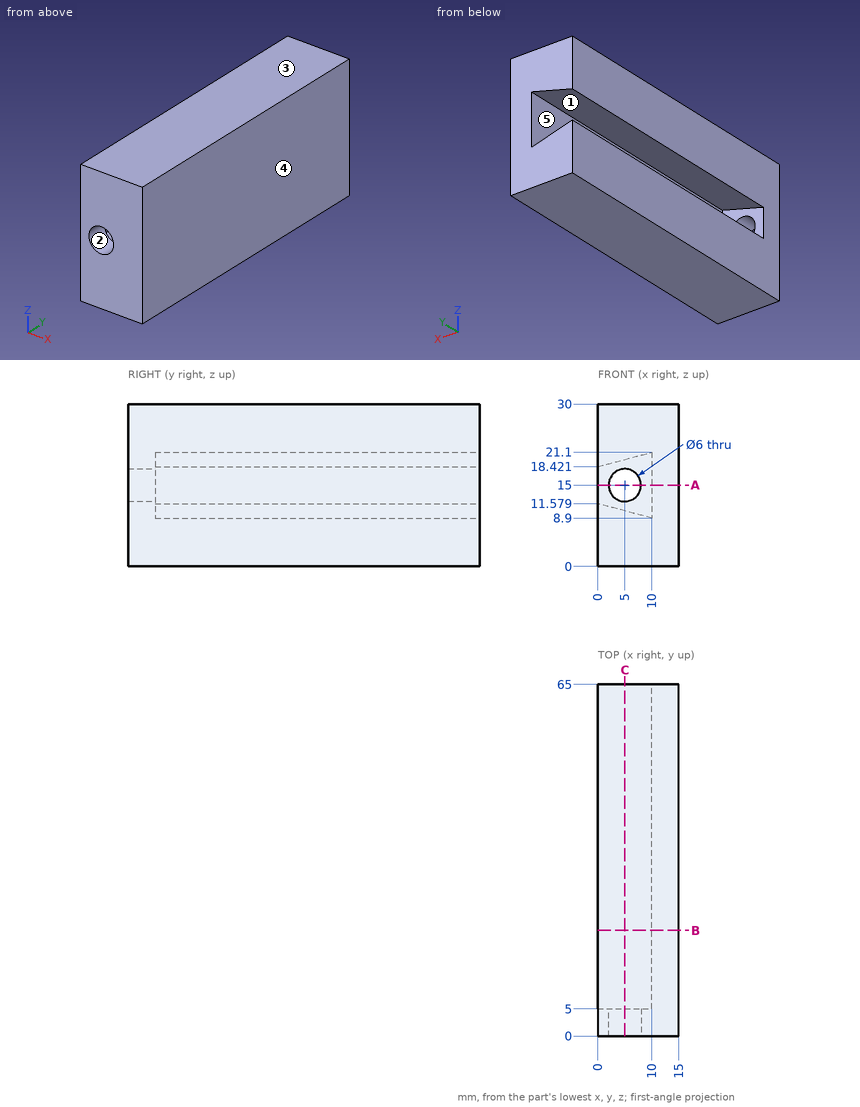
Study the drawing (mm; zero at the part's minimum x, y, z) and answer. A direction names the side the tool comes from. Give positions to 0.01 mm unless a question says otherwise; leave off trailing zeros. Write each loop counter-clockwise with the first axis right and the second up, starting at its lowest first coordinate (ties: lowest second). Pieces come first, ordered by that corner, then holes. Notation, with made-up numbers: (50, 88.5) -> (95, 88.5) arc R20 cw to (95, 126.5) -> close; hole circle Ø11 at (72.25, 85). An arc over 180 degrees is marked (long way). Write item = value, one per line.
Q1. A flat-ended cylindrical pin translates along its axis: pin 1 Ø8 at (y, z) = (49.5, 21.5) entering from -X. Find the tip coordinate at first contact, or state that the pin passes through.
Computed values:
pin_1 = 0
Q2. Section B-B on y = 19.5 is taken. Determine the outline of the cut face in (x, z), and give its area (3 significant figures).
Computed values:
outline = (0, 0) -> (15, 0) -> (15, 30) -> (0, 30) -> (0, 18.42) -> (10, 21.1) -> (10, 8.9) -> (0, 11.58) -> close
area = 355 mm^2
Q3. A tool of negligible diameter and unlimited length cuts with its end or side. For the marked faces 1 and 2, from which of +Z, -Z, +X, -X, +Y, -Y can it reach the whole face along a straight path? Write none if from no direction.
Computed values:
face_1 = +Y
face_2 = +Y, -Y
Q4. Section C-C on x = 5 is taken. Determine the outline of the cut face in (y, z).
Computed values:
outline = (0, 0) -> (65, 0) -> (65, 10.24) -> (5, 10.24) -> (5, 12) -> (0, 12) -> close; (0, 18) -> (5, 18) -> (5, 19.76) -> (65, 19.76) -> (65, 30) -> (0, 30) -> close
Q5. Consider line 1 along Z through (x, y) = (5, 1.65); line 2 along Z through (x, y) = (1.5, 9); line 3 along X through (y, z) = (31, 18.25). Determine where each line is inside the solid, lowest interval first.
Computed values:
line_1 = 0 to 12, 18 to 30
line_2 = 0 to 11.18, 18.82 to 30
line_3 = 10 to 15
Q6. For a pull along Z with two mould halves and no side action, classify the marked faces 3, 4 and 5 as pulls with the +Z half, pulls with the -Z half, needs draft (parallel to the pull), parting line crosses it, or undercut.
Computed values:
face_3 = pulls with the +Z half
face_4 = needs draft
face_5 = undercut
Q7. Section A-A on z = 15 is taken. Determine the outline of the cut face in (x, y).
Computed values:
outline = (0, 0) -> (2, 0) -> (2, 5) -> (0, 5) -> close; (8, 0) -> (15, 0) -> (15, 65) -> (10, 65) -> (10, 5) -> (8, 5) -> close
